Autodesk Inventor part; units mm, degrees
ref_plane "YZ Plane" through (0, 0, 0) normal (1, 0, 0) x (0, 1, 0)
ref_plane "XZ Plane" through (0, 0, 0) normal (0, 1, 0) x (-1, 0, 0)
ref_plane "XY Plane" through (0, 0, 0) normal (0, 0, 1) x (1, 0, 0)
sketch "Szkic1" plane through (0, 0, 0) normal (1, 0, 0) x (0, 1, 0)
  circle A0 centre (0, 0) radius 16
  dimension "d0" = 32
extrude "Wyciągnięcie proste1" add sketch "Szkic1" along normal blind 28
sketch "Szkic2" plane through (0, 0, 0) normal (-1, 0, 0) x (0, 0, 1)
  circle A0 centre (0, 0) radius 11.5
  dimension "d3" = 23
extrude "Wyciągnięcie proste2" cut sketch "Szkic2" against normal blind 30.8
sketch "Szkic3" plane through (0, 0, 0) normal (-1, 0, 0) x (0, 0, 1)
  circle A0 centre (0, 0) radius 16
extrude "Wyciągnięcie proste3" add sketch "Szkic3" against normal blind 2
sketch "Szkic4" plane through (0, 0, 0) normal (-1, 0, 0) x (0, 0, 1)
  circle A0 centre (0, 0) radius 1.8
  dimension "d8" = 3.6
extrude "Wyciągnięcie proste4" cut sketch "Szkic4" against normal blind 28
sketch "Szkic5" plane through (2, 0, 0) normal (1, 0, 0) x (0, 0, -1)
  circle A0 centre (0, 0) radius 1.8
  circle A1 centre (0, 0) radius 11.5
extrude "Wyciągnięcie proste5" add sketch "Szkic5" along normal blind 9
properties part number "kolo_tetsowe"
CAD build for the part. Positions are in the model's coordinates, mm. A direction names the side the tool comes from. Coordinates: 2 decimals unless noted, no trailing zeros. Order: outer loops, then holes, each group sorted by start corner. A loop starts at its lowest first (then second) coordinate and runs counter-clockwise, first axis right, second up.
(1) Mould opens along Y. For faces 1 (the face through (19.4, 11.4, -1.5)), 2 (the face through (13.8, -3.47, 15.62)), 3 (the face through (0, 0, -3)) say: released by +Y, released by -Y, zero draft, split by the parting line, or undercut.
Solution:
face 1: undercut
face 2: split by the parting line
face 3: zero draft
(2) Which spindle directions (+Z, -Z, +X, -X, +Y, -Y) get a long thin tool onto all of the face, cutting with end or side? Do faces 4 (the face through (11, -2, 0)), 5 (the face through (28, -11, 4)). Say none if no direction does.
Solution:
face 4: +X
face 5: +Z, -Z, +X, +Y, -Y
(3) Saw through at C-C, the plane x = 9.25. Write the cut outline in (y, z).
Solution:
outline: circle Ø32 at (0, 0); hole circle Ø3.6 at (0, 0)
(4) Saw through at A-A, the plane y = 0. Write the cut outline in (x, z), and give its area (3 significant figures).
Solution:
outline: (0, -16) - (28, -16) - (28, -11.5) - (11, -11.5) - (11, -1.8) - (0, -1.8) - close; (0, 1.8) - (11, 1.8) - (11, 11.5) - (28, 11.5) - (28, 16) - (0, 16) - close
area: 465 mm2
(5) Saw through at D-D, the plane z = 4. Write the cut outline in (x, y).
Solution:
outline: (0, -15.49) - (28, -15.49) - (28, -10.78) - (11, -10.78) - (11, 10.78) - (28, 10.78) - (28, 15.49) - (0, 15.49) - close
(6) Drill centre lines: L1, parallel to Z at x = 6, y = 0; L2, parallel to X at y = 5, z = -1.5; L3, parallel to Y at x = 22, z = 1. Where is each one in solid material? Low to high.
Solution:
L1: z = -16 to -1.8, 1.8 to 16
L2: x = 0 to 11
L3: y = -15.97 to -11.46, 11.46 to 15.97
(7) Pin check, flat tips, straight feed: pin 1 Ø5 at (x, z) = (15.5, 10) entering from +Y; pin 2 Ø1 at (x, z) = (22.5, 5.5) entering from -Y; pin 3 Ø4 at (x, y) = (20, -6) entering from -Z. Stop position of each tip, or through.
Solution:
pin 1: stops at y = 14.13
pin 2: stops at y = -15.2
pin 3: stops at z = -15.49
